Autodesk Inventor part; units mm, degrees
ref_plane "YZ Plane" through (0, 0, 0) normal (1, 0, 0) x (0, 1, 0)
ref_plane "XZ Plane" through (0, 0, 0) normal (0, 1, 0) x (-1, 0, 0)
ref_plane "XY Plane" through (0, 0, 0) normal (0, 0, 1) x (1, 0, 0)
sketch "スケッチ1" plane through (0, 0, 0) normal (0, 0, 1) x (1, 0, 0)
  line L0 (0, 0) -> (42.6795, 0)
  line L1 (2.6795, -10) -> (42.6795, -10)
  line L2 (42.6795, 0) -> (42.6795, -10)
  line L3 (2.6795, -10) -> (-83.923, -60)
  line L4 (-80.2628, -46.3397) -> (0, 0)
  line L5 (-83.923, -60) -> (-93.923, -42.6795)
  line L6 (-93.923, -42.6795) -> (-85.2628, -37.6795)
  line L7 (-85.2628, -37.6795) -> (-80.2628, -46.3397)
  point P0 (-88.923, -51.3397)
  dimension "d1" = 40
  dimension "d2" = 10
  dimension "d3" = 100
  dimension "d4" = 150
  dimension "d5" = 10
  dimension "d6" = 20
  dimension "d7" = 10
  dimension "d8" = 10
  dimension "d9" = 10
extrude "押し出し1" add sketch "スケッチ1" along normal mid plane 5
sketch "スケッチ2" plane through (0, 0, 2.5) normal (0, 0, 1) x (1, 0, 0)
  line L0 (36.4795, -7.1) -> (39.6795, -7.1)
  line L1 (39.6795, -7.1) -> (39.6795, -2.9)
  line L2 (39.6795, -2.9) -> (36.4795, -2.9)
  line L3 (36.4795, -2.9) -> (36.4795, -7.1)
  line L4 (36.4795, -7.1) -> (39.6795, -2.9) construction
  line L5 (39.6795, -7.1) -> (36.4795, -2.9) construction
  line L6 (42.6795, 0) -> (0, 0)
  line L7 (2.6795, -10) -> (42.6795, -10)
  line L8 (42.6795, -10) -> (42.6795, 0)
  point P0 (38.0795, -5)
  dimension "d14" = 3
  dimension "d15" = 3.2
  dimension "d41" = 4.2
  dimension "d42" = 2.9
extrude "押し出し2" cut sketch "スケッチ2" against normal blind 5
sketch "スケッチ3" plane through (0, 0, 2.5) normal (0, 0, 1) x (1, 0, 0)
  line L0 (-83.923, -60) -> (2.6795, -10)
  line L1 (-85.2628, -37.6795) -> (-93.923, -42.6795)
  line L2 (-80.2628, -46.3397) -> (-85.2628, -37.6795)
  line L3 (-93.923, -42.6795) -> (-83.923, -60)
  point P0 (0, 0)
  point P1 (-87.0929, -44.5096)
  point P2 (-82.0929, -53.1699)
  point P3 (-47.4519, -33.1699)
  dimension "d18" = 5
  dimension "d19" = 5
  dimension "d20" = 5
  dimension "d21" = 5
  dimension "d22" = 5
  dimension "d23" = 40
hole "穴1" at (-82.0929, -53.1699, 2.5) at (-47.4519, -33.1699, 2.5) direction (0, 0, -1) diameter 4.5 end through all
fillet "フィレット1" radius 2 8 edges at (0, 0, 0) (2.6795, -10, 0) (42.6795, 0, 0) (42.6795, -10, 0) (-80.2628, -46.3397, 0) (-85.2628, -37.6795, 0) (-93.923, -42.6795, 0) (-83.923, -60, 0)
sketch "スケッチ4" plane through (0, 0, 2.5) normal (0, 0, 1) x (1, 0, 0)
  arc A0 (-84.923, -58.2679) -> (-82.191, -59) centre (-83.191, -57.2679) ccw
  line L0 (-82.191, -59) -> (2.2154, -10.2679)
  arc A1 (3.2154, -10) -> (2.2154, -10.2679) centre (3.2154, -12) ccw
  line L1 (3.2154, -10) -> (40.6795, -10)
  arc A2 (40.6795, -10) -> (42.6795, -8) centre (40.6795, -8) ccw
  line L2 (42.6795, -8) -> (42.6795, -2)
  arc A3 (42.6795, -2) -> (40.6795, 0) centre (40.6795, -2) ccw
  line L3 (40.6795, 0) -> (0.5359, 0)
  arc A4 (0.5359, 0) -> (-0.4641, -0.2679) centre (0.5359, -2) ccw
  line L4 (-0.4641, -0.2679) -> (-78.5307, -45.3397)
  arc A5 (-81.2628, -44.6077) -> (-78.5307, -45.3397) centre (-79.5307, -43.6077) ccw
  line L5 (-81.2628, -44.6077) -> (-84.2628, -39.4115)
  arc A6 (-84.2628, -39.4115) -> (-86.9948, -38.6795) centre (-85.9948, -40.4115) ccw
  line L6 (-86.9948, -38.6795) -> (-92.191, -41.6795)
  arc A7 (-92.191, -41.6795) -> (-92.923, -44.4115) centre (-91.191, -43.4115) ccw
  line L7 (-92.923, -44.4115) -> (-84.923, -58.2679)
  circle A8 centre (-47.4519, -33.1699) radius 2.25
  circle A9 centre (-82.0929, -53.1699) radius 2.25
  line L8 (36.4795, -2.9) -> (39.6795, -2.9)
  line L9 (39.6795, -2.9) -> (39.6795, -7.1)
  line L10 (39.6795, -7.1) -> (36.4795, -7.1)
  line L11 (36.4795, -7.1) -> (36.4795, -2.9)
  point P0 (0, 0)
  point P1 (-87.0929, -44.5096)
  dimension "d32" = 5
  dimension "d33" = 5
hole "穴2" at (-87.0929, -44.5096, 2.5) direction (0, 0, -1) diameter 3.3 end through all
properties part number "刃固定パーツ"
Can you work these out from the model? Positions are in its coordinate system, mm. A direction names the side the tool comes from. Round coordinates to 2 decimals unless told otherwise and drop trailing zeros. Loops run counter-clockwise (first coordinate to the right, second up) from the corner with the lowest first, then second, coordinate; pieces in that order, holes last. Notation, with made-up numbers: (72, 40.25) - (77, 40.25) arc R26 cw to (77, 76.25) - close; hole circle Ø1 at (-34, 74). An arc over 180 degrees is marked (long way). Answer in a Markdown table with one row per item. Add a question column.
Q1. I want a section at B-B on z = -1.3. List the corners of the cut face in (x, y) for me, and give its area (3 significant figures).
Q2. For pin 1 Ø1.5 at (y, z) = (-27, -1) entering from +X; pin 2 Ø2.5 at (x, y) = (-87.09, -44.51) entering from -Z; pin 3 Ø1.5 at (x, z) = (15.5, 0) entering from -Y; pin 4 Ø2 at (y, z) = (-4.5, 0.5) entering from -X, each with a flat end and sliding along its axis, tell me the tip position at first contact or that it passes through.
Q3. I want a section at D-D on y = -19.5. List the corners of the cut face in (x, z) for me.
Q4. I need wall thicknesses on L1, parallel to X at y = -45, z = -0.6; L2, parallel to X at y = -41.5, z = -1.15; L3, parallel to Y at x = 32, z = 0.95. Which ranges of each line are inside material? Lowest first, please.
Q5. I want a section at C-C on x = -58. List the corners of the cut face in (y, z) for me.
Q6. Which directions (+Z, -Z, +X, -X, +Y, -Y) give clear straight access to the entire face, cutting with the end or side of a thin tool? Please do faces 1 (the flat face through (38, -7.1, 0)), 2 (the flat face through (-82.784, -41.973, -0.035)), 3 (the flat face through (22, -10, 0)), 4 (the cylindrical face through (-83.687, -59.205, -0.035)), 5 (the flat face through (-88.867, -51.437, -0.035)).
Q7. We'd pull the mould along Y, two halves only. Please class faces 6 (the flat face through (-26, -23, 2.5)), 7 (the flat face through (39.68, -5, 0)), 8 (the flat face through (38, -2.9, 0)), 9 (the flat face through (-89.63, -40.2, -0.04)): pulls with the +Y half, pulls with the -Y half, needs draft (parallel to the pull), parting line crosses it, or undercut.
Q8. I want a section at A-A on y = -34. List the corners of the cut face in (x, z) for me.
A:
| question | item | result |
|---|---|---|
| 1 | outline | (-92.92, -44.41) - (-84.92, -58.27) arc R2 ccw to (-82.19, -59) - (2.22, -10.27) arc R2 cw to (3.22, -10) - (40.68, -10) arc R2 ccw to (42.68, -8) - (42.68, -2) arc R2 ccw to (40.68, 0) - (0.54, 0) arc R2 ccw to (-0.46, -0.27) - (-78.53, -45.34) arc R2 cw to (-81.26, -44.61) - (-84.26, -39.41) arc R2 ccw to (-86.99, -38.68) - (-92.19, -41.68) arc R2 ccw to start; hole circle Ø3.3 at (-87.09, -44.51); hole circle Ø4.5 at (-82.09, -53.17); hole circle Ø4.5 at (-47.45, -33.17); hole (36.48, -7.1) - (39.68, -7.1) - (39.68, -2.9) - (36.48, -2.9) - close |
| 1 | area | 1,470 mm^2 |
| 2 | pin 1 | x = -25.47 |
| 2 | pin 2 | through |
| 2 | pin 3 | y = -10 |
| 2 | pin 4 | x = -9.53 |
| 3 | outline | (-33.78, -2.5) - (-13.77, -2.5) - (-13.77, 2.5) - (-33.78, 2.5) - close |
| 4 | L1 | -92.58 to -88.67, -85.52 to -80.97, -77.94 to -57.94 |
| 4 | L2 | -91.88 to -83.06, -71.88 to -51.88 |
| 4 | L3 | -10 to 0 |
| 5 | outline | (-45.03, -2.5) - (-33.49, -2.5) - (-33.49, 2.5) - (-45.03, 2.5) - close |
| 6 | face 1 | +Z, -Z |
| 6 | face 2 | +Z, -Z, +Y |
| 6 | face 3 | +Z, -Z, +X, -Y |
| 6 | face 4 | +Z, -Z, -Y |
| 6 | face 5 | +Z, -Z, -X, -Y |
| 7 | face 6 | needs draft |
| 7 | face 7 | undercut |
| 7 | face 8 | undercut |
| 7 | face 9 | pulls with the +Y half |
| 8 | outline | (-58.89, -2.5) - (-49.54, -2.5) - (-49.54, 2.5) - (-58.89, 2.5) - close; (-45.36, -2.5) - (-38.89, -2.5) - (-38.89, 2.5) - (-45.36, 2.5) - close |
